Part print with two shaded views. Sizes in mm from the minimum x, y, z corner. A direction names the side the tool comes from. Coordinates: 2 decimals unless noted, no trailing zeros. Loops run counter-clockwise (first coordinate to the right, second up) from the corner with the lowest first, then second, coordinate; pieces in that order, holes last.
Item 1: Drill centre lines: line 1 along Z through (x, y) = (11, 0.1); line 2 along X through (y, z) = (5, 11). Where is each one in solid material? Low to high.
Item 2: 3-axis set-ups, long thin cutter, end or side, ignore diameter. For the marked faces 5 and 6: which of +Z, -Z, +X, -X, +Y, -Y reach the whole face in a straight line?
Item 3: Mould opens along Z. For the marked faces 1, 2, 3 and 4 say: released by +Z, released by -Z, zero draft, split by the parting line, or undercut.
Item 4: Flat gauge pin, fed straight in: pin 1 (3 mm diameter, centred on x = 3, y = 1.5, fed in from +Z). Where does the tip first touch, or does it go through?
Item 5: Cut at B-B (x = 11). List the corners of the cut face in (y, z).
Item 6: Cut at A-A (z = 11). List the corners of the cut face in (x, y).
Item 7: Cut at D-D (z = 3). List the corners of the cut face in (x, y).
Item 8: Cut at C-C (y = 1.25). List the corners of the cut face in (x, z), and give its area (3 significant figures).
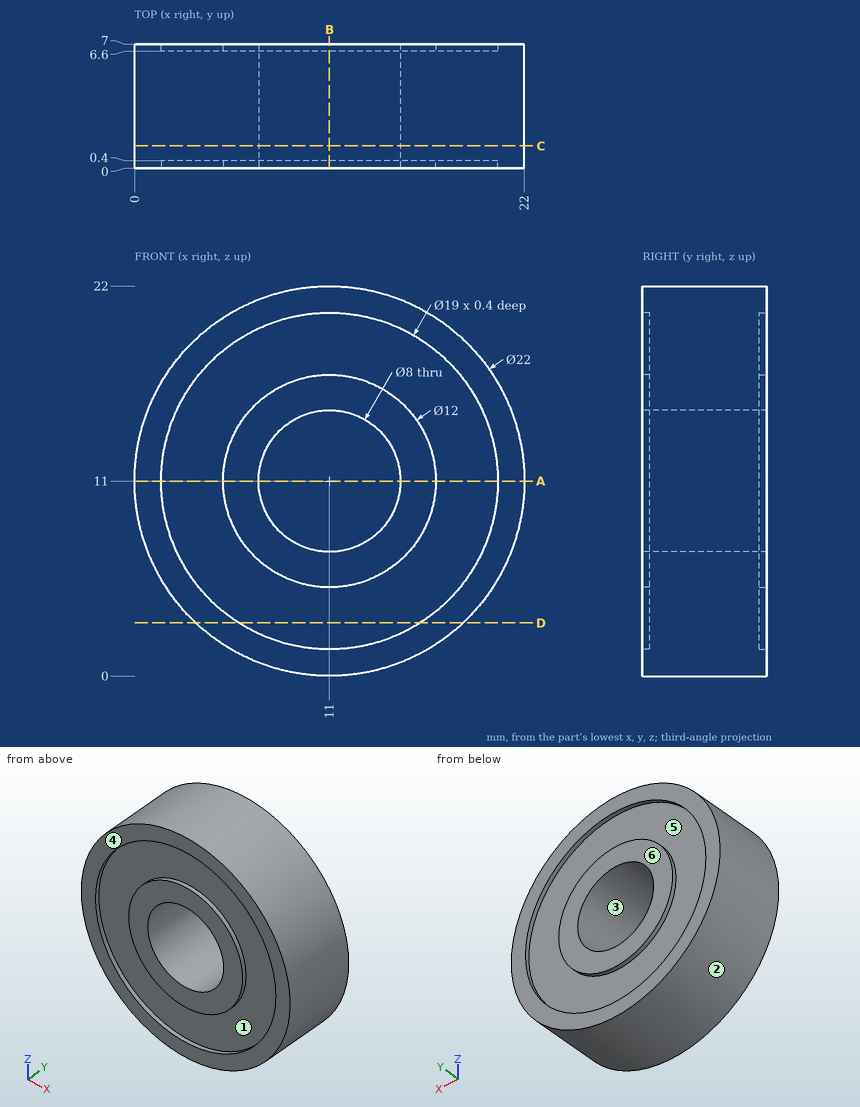
Filled sheet:
1. line 1: z = 0 to 1.5, 5 to 7, 15 to 17, 20.5 to 22
1. line 2: x = 0 to 7, 15 to 22
2. face 5: +Y
2. face 6: +Z, -Z, +X, -X, +Y
3. face 1: undercut
3. face 2: split by the parting line
3. face 3: undercut
3. face 4: zero draft
4. pin 1: stops at z = 19.87
5. outline: (0, 0) - (7, 0) - (7, 1.5) - (6.6, 1.5) - (6.6, 5) - (7, 5) - (7, 7) - (0, 7) - (0, 5) - (0.4, 5) - (0.4, 1.5) - (0, 1.5) - close; (0, 15) - (7, 15) - (7, 17) - (6.6, 17) - (6.6, 20.5) - (7, 20.5) - (7, 22) - (0, 22) - (0, 20.5) - (0.4, 20.5) - (0.4, 17) - (0, 17) - close
6. outline: (0, 0) - (1.5, 0) - (1.5, 0.4) - (5, 0.4) - (5, 0) - (7, 0) - (7, 7) - (5, 7) - (5, 6.6) - (1.5, 6.6) - (1.5, 7) - (0, 7) - close; (15, 0) - (17, 0) - (17, 0.4) - (20.5, 0.4) - (20.5, 0) - (22, 0) - (22, 7) - (20.5, 7) - (20.5, 6.6) - (17, 6.6) - (17, 7) - (15, 7) - close
7. outline: (3.45, 0) - (5.88, 0) - (5.88, 0.4) - (16.12, 0.4) - (16.12, 0) - (18.55, 0) - (18.55, 7) - (16.12, 7) - (16.12, 6.6) - (5.88, 6.6) - (5.88, 7) - (3.45, 7) - close
8. outline: circle Ø22 at (11, 11); hole circle Ø8 at (11, 11)
8. area: 330 mm2
